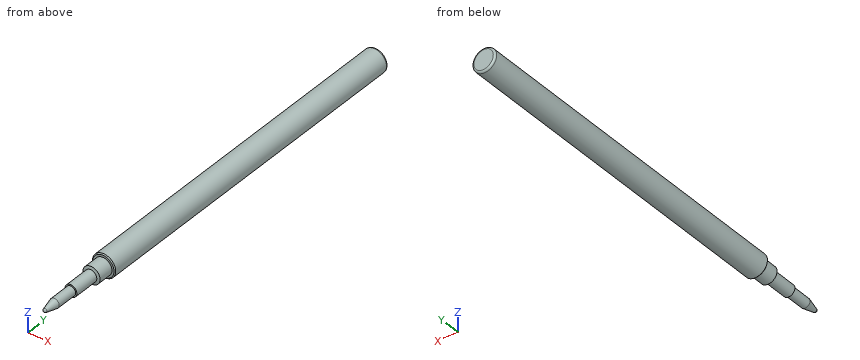
from build123d import *

# Parameters (mm, degrees)
F0_W    = 90.932
F0_H    = 3.0861
F4_SIZE = 0.254
F5_R    = 0.508


with BuildPart() as f1:
    # F0 (on Right) → F1 (revolve)
    with BuildSketch(Plane.YZ):
        with Locations((-5.334, 1.54305)):
            Rectangle(F0_W, F0_H)
    revolve(axis=Axis((0, -5.334, 0), (0, 1, 0)))

    # F2 (on Right) → F3 (revolve)
    with BuildSketch(Plane.YZ):
        with BuildLine():
            Line((-70.612, 0), (-50.8, 0))
            Line((-50.8, 0), (-50.8, 1.2446))
            Line((-50.8, 1.2446), (-50.8, 2.286))
            Line((-50.8, 2.286), (-54.7624, 2.286))
            Line((-54.7624, 2.286), (-54.970556, 1.5748))
            Line((-54.970556, 1.5748), (-61.595, 1.5748))
            Line((-61.595, 1.5748), (-61.595, 1.2446))
            Line((-61.595, 1.2446), (-67.056, 1.2446))
            Line((-67.056, 1.2446), (-70.221173, 0.494302))
            ThreePointArc((-70.221173, 0.494302), (-70.50249, 0.315071), (-70.612, 0))
        make_face()
    revolve(axis=Axis((0, -60.706, 0), (0, -1, 0)))

    # F4
    f4_edges = [f1.edges().sort_by_distance(p)[0] for p in [
        (0, -50.8, -3.0861),
    ]]
    chamfer(f4_edges, length=F4_SIZE)

    # F5
    f5_edges = [f1.edges().sort_by_distance(p)[0] for p in [
        (0, 40.132, -3.0861),
    ]]
    fillet(f5_edges, radius=F5_R)


solid = f1.part
Geometry: final body of the model. Coordinates: model frame, mm. Coordinates: 2 decimals unless noted, no trailing zeros. Loops run counter-clockwise (first coordinate to the right, second up) from the corner with the lowest first, then second, coordinate; pieces in that order, holes last. Notation, with made-up numbers: (76, 0.5) - (124, 0.5) arc R14 cw to (124, 26.5) - close; hole circle Ø6 at (-15, 1). An arc over 180 degrees is marked (long way). Put each result on its own line as item: value. Start each with the question number.
Q1. Line query: line 1 (Y direction, x = 2.25, z = 0.75); line 2 (Z direction, x = -1.25, y = -31.5). Output: solid intervals per line, ascending.
Q2. Cut plane A-A, the plane y = -59.5. Return loops of the section in (x, z).
Q3. Cut plane B-B, the plane y = 25.5. Return loops of the section in (x, z).
Q4. Pin query (flat end, axial travel): pin 1 Ø3 at (y, z) = (-17.5, -2) entering from -X; pin 2 Ø1.5 at (x, z) = (-0.5, -2) entering from -Y (3 decimals); pin 3 Ø1.7 at (x, z) = (-1, -0.5) entering from -Y. Return the tip coordinate at first contact, or that it passes through.
Filled sheet:
1. line 1: -50.8 to 40.13
1. line 2: -2.82 to 2.82
2. outline: circle Ø3.15 at (0, 0)
3. outline: circle Ø6.17 at (0, 0)
4. pin 1: x = -3.05
4. pin 2: y = -61.595
4. pin 3: y = -70.54
